from build123d import *

# Parameters (mm, degrees)
BOSS_EXTRUDE1_DEPTH = 5
CUT_EXTRUDE1_REACH  = 55.66
SKETCH2_R           = 1.51


with BuildPart() as part:
    # Sketch1 → Boss-Extrude1 (new body)
    with BuildSketch(Plane(origin=(0, 0, 0), x_dir=(1, 0, 0), z_dir=(0, 1, 0))):
        with BuildLine():
            ThreePointArc((0, 10), (-10, 0), (0, -10))
            Line((0, -10), (45.601011206, -6.227938292))
            ThreePointArc((45.601011206, -6.227938292), (52.479923025, 1.451771759), (45.191159304, 8.743636932))
            Line((45.191159304, 8.743636932), (0, 10))
        make_face()
    extrude(amount=BOSS_EXTRUDE1_DEPTH)

    # Sketch2 → Cut-Extrude1 (cut, up to next)
    with BuildSketch(Plane(origin=(0, 5, 0), x_dir=(1, 0, 0), z_dir=(0, 1, 0)), mode=Mode.PRIVATE) as cut_extrude1_sk1:
        with Locations(Location((0, 0, 0), (0, 0, 270))):
            Circle(SKETCH2_R)
    cut_extrude1_tool1 = extrude(cut_extrude1_sk1.sketch, amount=-CUT_EXTRUDE1_REACH, mode=Mode.PRIVATE) & part.part
    # Sketch2 → Cut-Extrude1 (cut, up to next)
    with BuildSketch(Plane(origin=(0, 5, 0), x_dir=(1, 0, 0), z_dir=(0, 1, 0)), mode=Mode.PRIVATE) as cut_extrude1_sk2:
        with Locations(Location((44.98273173, 1.246533628, 0), (0, 0, 270))):
            Circle(SKETCH2_R)
    cut_extrude1_tool2 = extrude(cut_extrude1_sk2.sketch, amount=-CUT_EXTRUDE1_REACH, mode=Mode.PRIVATE) & part.part
    add(cut_extrude1_tool1.solids().sort_by_distance((0, 5, 0))[0], mode=Mode.SUBTRACT)
    add(cut_extrude1_tool2.solids().sort_by_distance((44.982732, 5, -1.246534))[0], mode=Mode.SUBTRACT)


solid = part.part
Can you work these out from the model? Positions are in its coordinate system, mm. Give positions to 0.01 mm unless a question says otherwise; leave off trailing zeros. Write each loop counter-clockwise with the first axis right and the second up, starting at its lowest first coordinate (ties: lowest second). Pieces come first, ordered by that corner, then holes. Notation, with made-up numbers: M -37,15.5 L -8,15.5 A22 cw -8,43.5 Z; hole C -9,0.25 d2. An arc over 180 degrees is marked long. Answer in a Markdown table with one row per item. Add a question column.
Item 1: Imagine slicing it at A-A, the plane y = 3.6. Write out the boundary of the cut face in (x, z).
Item 2: We'd pull the mould along X, two halves only. Please class faces 1 (the flat face through (21, 0, 0)), 2 (the cylindrical face through (43.509, 2.535, -1.574)), 3 (the cylindrical face through (52.483, 2.465, -1.293)), 4 (the cylindrical face through (1.497, 2.535, -0.197)): released by +X, released by -X, zero draft, split by the parting line, or undercut.
Item 3: Please list where these lines run through material, in increasing order: L1, parallel to X at y = 1.25, z = 0; L2, parallel to Z at x = 45.5, y = 1.6; L3, parallel to Z at x = 46, y = 2.
Item 4: Imagine slicing it at B-B, the plane x = -5. Write out the boundary of the cut face in (y, z).
Item 5: For pin 1 Ø3 at (x, z) = (45, 6.5) entering from +Y; pin 2 Ø1 at (y, z) = (1, -3) entering from +X; pin 3 Ø2.5 at (x, z) = (44.98, -1.25) entering from +Y, each with a flat end and sliding along its axis, tell me the tip position at first contact or that it passes through.
Item 6: Imagine slicing it at C-C, the plane z = -6.5. Write out the boundary of the cut face in (x, y), plus the area to 3 significant figures.
Evaluation:
| question | item | result |
|---|---|---|
| 1 | outline | M 0,-10 L 45.19,-8.74 A7.5 ccw 45.6,6.23 L 0,10 A10 ccw Z; hole C 0,0 d3.02; hole C 44.98,-1.25 d3.02 |
| 2 | face 1 | zero draft |
| 2 | face 2 | undercut |
| 2 | face 3 | released by +X |
| 2 | face 4 | undercut |
| 3 | L1 | x = -10 to -1.51, 1.51 to 44.13, 45.83 to 52.38 |
| 3 | L2 | z = -8.73 to -2.67, 0.17 to 6.24 |
| 3 | L3 | z = -8.68 to -2.36, -0.13 to 6.18 |
| 4 | outline | M 0,-8.66 L 5,-8.66 L 5,8.66 L 0,8.66 Z |
| 5 | pin 1 | stops at y = 5 |
| 5 | pin 2 | stops at x = 52.38 |
| 5 | pin 3 | passes through |
| 6 | outline | M -7.6,0 L 50.34,0 L 50.34,5 L -7.6,5 Z |
| 6 | area | 290 mm² |
